```python
from build123d import *

# Parameters (mm, degrees)
SKETCH1_W               = 107.95
SKETCH1_H               = 85.725
BOSS_EXTRUDE1_DEPTH     = 2.54
SKETCH2_W               = 107.95
SKETCH2_H               = 85.725
SKETCH2_W_2             = 104.775
SKETCH2_H_2             = 82.55
BOSS_EXTRUDE2_DEPTH     = 25.4
SKETCH3_R               = 3.175
CUT_EXTRUDE1_DEPTH      = 141.650708228
CUT_EXTRUDE1_DEPTH_BACK = 141.650708228
SKETCH4_R               = 3.175
CUT_EXTRUDE2_DEPTH      = 141.650708228
CUT_EXTRUDE2_DEPTH_BACK = 141.650708228
SKETCH5_W               = 21.844
SKETCH5_H               = 44.45
BOSS_EXTRUDE3_DEPTH     = 1.5875
SKETCH6_W               = 2.54
SKETCH6_H               = 44.45
BOSS_EXTRUDE4_DEPTH     = 12.7
SKETCH7_R               = 6.35
BOSS_EXTRUDE5_DEPTH     = 6.35
SKETCH8_R               = 6.35
BOSS_EXTRUDE6_DEPTH     = 6.35
FILLET1_R               = 2.54
FILLET2_R               = 2.54
SKETCH9_R               = 6.35
BOSS_EXTRUDE7_DEPTH     = 6.35
SKETCH10_R              = 6.35
BOSS_EXTRUDE8_DEPTH     = 6.35
FILLET3_R               = 2.54
SKETCH11_R              = 3.175
CUT_EXTRUDE4_DEPTH      = 145.608615667
CUT_EXTRUDE4_DEPTH_BACK = 145.608615667
SKETCH12_R              = 3.175
CUT_EXTRUDE5_DEPTH      = 145.608615667
CUT_EXTRUDE5_DEPTH_BACK = 145.608615667


with BuildPart() as part:
    # Sketch1 → Boss-Extrude1 (new body)
    with BuildSketch(Plane(origin=(0, 0, 0), x_dir=(1, 0, 0), z_dir=(0, 1, 0))):
        with Locations((53.975, 42.8625)):
            Rectangle(SKETCH1_W, SKETCH1_H)
    extrude(amount=BOSS_EXTRUDE1_DEPTH)

    # Sketch2 → Boss-Extrude2 (add)
    with BuildSketch(Plane(origin=(0, 2.54, 0), x_dir=(1, 0, 0), z_dir=(0, 1, 0))):
        with Locations((53.975, 42.8625)):
            Rectangle(SKETCH2_W, SKETCH2_H)
        with Locations((53.975, 42.8625)):
            Rectangle(SKETCH2_W_2, SKETCH2_H_2, mode=Mode.SUBTRACT)
    extrude(amount=BOSS_EXTRUDE2_DEPTH)

    # Sketch3 → Cut-Extrude1 (cut, two sides)
    with BuildSketch(Plane(origin=(0, 0, -85.725), x_dir=(-1, 0, 0), z_dir=(0, 0, -1))) as cut_extrude1_sk:
        with Locations((-11.1125, 14.028153998)):
            Circle(SKETCH3_R)
    extrude(amount=CUT_EXTRUDE1_DEPTH, mode=Mode.SUBTRACT)
    extrude(cut_extrude1_sk.sketch, amount=-CUT_EXTRUDE1_DEPTH_BACK, mode=Mode.SUBTRACT)

    # Sketch4 → Cut-Extrude2 (cut, two sides)
    with BuildSketch(Plane(origin=(0, 0, -85.725), x_dir=(-1, 0, 0), z_dir=(0, 0, -1))) as cut_extrude2_sk:
        with Locations((-94.9325, 12.514694303)):
            Circle(SKETCH4_R)
    extrude(amount=CUT_EXTRUDE2_DEPTH, mode=Mode.SUBTRACT)
    extrude(cut_extrude2_sk.sketch, amount=-CUT_EXTRUDE2_DEPTH_BACK, mode=Mode.SUBTRACT)

    # Sketch5 → Boss-Extrude3 (add)
    with BuildSketch(Plane(origin=(0, 2.54, 0), x_dir=(1, 0, 0), z_dir=(0, 1, 0))):
        with Locations((12.5095, 42.8625)):
            Rectangle(SKETCH5_W, SKETCH5_H)
    extrude(amount=BOSS_EXTRUDE3_DEPTH)

    # Sketch6 → Boss-Extrude4 (add)
    with BuildSketch(Plane(origin=(0, 4.1275, 0), x_dir=(1, 0, 0), z_dir=(0, 1, 0))):
        with Locations((22.1615, 42.8625)):
            Rectangle(SKETCH6_W, SKETCH6_H)
    extrude(amount=BOSS_EXTRUDE4_DEPTH)

    # Sketch7 → Boss-Extrude5 (add)
    with BuildSketch(Plane.XY):
        with Locations(Location((11.1125, 14.028153998, 0), (0, 0, 180))):
            Circle(SKETCH7_R)
    extrude(amount=BOSS_EXTRUDE5_DEPTH)

    # Sketch8 → Boss-Extrude6 (add)
    with BuildSketch(Plane.XY):
        with Locations(Location((94.9325, 12.514694303, 0), (0, 0, 180))):
            Circle(SKETCH8_R)
    extrude(amount=BOSS_EXTRUDE6_DEPTH)

    # Fillet1
    fillet1_edges = [part.edges().sort_by_distance(p)[0] for p in [
        (17.4625, 14.028153998, 0),
    ]]
    fillet(fillet1_edges, radius=FILLET1_R)

    # Fillet2
    fillet2_edges = [part.edges().sort_by_distance(p)[0] for p in [
        (101.2825, 12.514694303, 0),
    ]]
    fillet(fillet2_edges, radius=FILLET2_R)

    # Sketch9 → Boss-Extrude7 (add)
    with BuildSketch(Plane(origin=(0, 0, -85.725), x_dir=(-1, 0, 0), z_dir=(0, 0, -1))):
        with Locations((-94.9325, 12.514694303)):
            Circle(SKETCH9_R)
    extrude(amount=BOSS_EXTRUDE7_DEPTH)

    # Sketch10 → Boss-Extrude8 (add)
    with BuildSketch(Plane(origin=(0, 0, -85.725), x_dir=(-1, 0, 0), z_dir=(0, 0, -1))):
        with Locations((-11.1125, 14.028153998)):
            Circle(SKETCH10_R)
    extrude(amount=BOSS_EXTRUDE8_DEPTH)

    # Fillet3
    fillet3_edges = [part.edges().sort_by_distance(p)[0] for p in [
        (101.2825, 12.514694303, -85.725),
        (17.4625, 14.028153998, -85.725),
    ]]
    fillet(fillet3_edges, radius=FILLET3_R)

    # Sketch11 → Cut-Extrude4 (cut, two sides)
    with BuildSketch(Plane.XY.offset(-85.725)) as cut_extrude4_sk:
        with Locations(Location((94.9325, 12.514694303, 0), (0, 0, 180))):
            Circle(SKETCH11_R)
    extrude(amount=CUT_EXTRUDE4_DEPTH, mode=Mode.SUBTRACT)
    extrude(cut_extrude4_sk.sketch, amount=-CUT_EXTRUDE4_DEPTH_BACK, mode=Mode.SUBTRACT)

    # Sketch12 → Cut-Extrude5 (cut, two sides)
    with BuildSketch(Plane.XY.offset(-85.725)) as cut_extrude5_sk:
        with Locations(Location((11.1125, 14.028153998, 0), (0, 0, 180))):
            Circle(SKETCH12_R)
    extrude(amount=CUT_EXTRUDE5_DEPTH, mode=Mode.SUBTRACT)
    extrude(cut_extrude5_sk.sketch, amount=-CUT_EXTRUDE5_DEPTH_BACK, mode=Mode.SUBTRACT)


solid = part.part
```
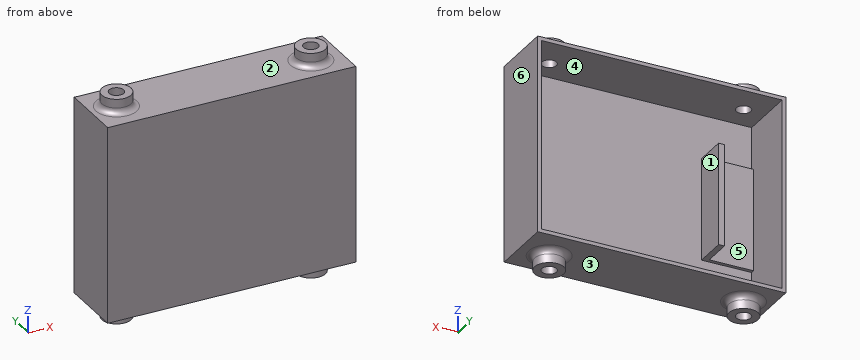
Check sheet for the modelled part. Datum: model origin and axes. Units: mm. Face numbers are marked on the shaded views. A direction names the side the tool comes from. Give positions to 0.01 mm unless a question says otherwise; leave off trailing zeros. Order: outer loops, then holes, each group sorted by start corner. A loop starts at its lowest first (then second) coordinate and runs counter-clockwise, first axis right, second up. Notation, with made-up numbers: (48, 0.25) -> (106, 0.25) arc R31 ccw to (106, 29.25) -> close; hole circle Ø3 at (1.25, 53). An arc over 180 degrees is marked (long way). Return JSON: item names as keys, results as strings.
1. Mould release check, pull along Z, two halves, no side actions. Record for the marked faces 1, 2, 3 and 4: +Z half, -Z half, draft (parallel to the pull), parting line (faces both ways), or undercut.
From the geometry:
{"face 1": "undercut", "face 2": "+Z half", "face 3": "-Z half", "face 4": "undercut"}
2. Go/stop test with flat-tipped pins: P1, Ø5, axis at x = 11.11, y = 14.03, coming from the +Z side; P2, Ø10, axis at x = 44, y = 15.5, coming from the -Z side (3 decimals); P3, Ø4, axis at x = 11, y = 5, coming from the +Z side; P4, Ø1.3, axis at x = 22.5, z = -44, coming from the +Y side. Record where each tip stops, or that it passes through.
From the geometry:
{"P1": "through", "P2": "z = -85.725", "P3": "z = 0.81", "P4": "y = 16.83"}
3. Cross-section at C-C, the plane z = -47. Record the cut outline in (x, y).
From the geometry:
{"outline": "(0, 0) -> (107.95, 0) -> (107.95, 27.94) -> (106.36, 27.94) -> (106.36, 2.54) -> (23.43, 2.54) -> (23.43, 16.83) -> (20.89, 16.83) -> (20.89, 4.13) -> (1.59, 4.13) -> (1.59, 27.94) -> (0, 27.94) -> close"}
4. Cross-section at D-D, the plane x = 13. Count the separate pieces of the cut face and the enclosed holes in it, plus the area to 3 significant figures.
From the geometry:
{"separate pieces": "3", "enclosed holes": "0", "area": "448 mm^2"}
5. Material ranges on probe 1 along X at (y, z) = (8.5, -29); probe 2 along X at (y, z) = (14, -9); probe 3 along Z at (x, y) = (86.5, 18.75) (1 decimal), recorded low to high. Write a range as [from, to].
From the geometry:
{"probe 1": "[0, 1.59], [20.89, 23.43], [106.36, 107.95]", "probe 2": "[0, 1.59], [106.36, 107.95]", "probe 3": "[-85.7, -84.1], [-1.6, 0]"}
6. Cross-section at B-B, the plane x = 61.5. Record the cut outline in (y, z) (1 decimal).
From the geometry:
{"outline": "(0, -85.7) -> (27.9, -85.7) -> (27.9, -84.1) -> (2.5, -84.1) -> (2.5, -1.6) -> (27.9, -1.6) -> (27.9, 0) -> (0, 0) -> close"}
7. Set-up check for the marked faces 5 and 6: record each of +Z, -Z, +X, -X, +Y, -Y from which the full face is reachable in a straight line by a thin tool's end or side.
From the geometry:
{"face 5": "+Y", "face 6": "+Z, -Z, +X, +Y, -Y"}
